The model under review builds one solid part; all positions refer to its coordinate system, in mm. Face numbers are marked on the shaded views. A direction names the side the tool comes from. Give positions to 0.01 mm unless a question says otherwise; leave off trailing zeros. Order: outer loops, then holes, each group sorted by start corner. A loop starts at its lowest first (then second) coordinate and runs counter-clockwise, first axis right, second up. Notation, with made-up numbers: (38.5, -9) -> (68.5, -9) arc R31 ccw to (68.5, 21) -> close; hole circle Ø10 at (-1.75, -16). An arc over 180 degrees is marked (long way). Use one line per item in the form item = value.
```python
from build123d import *

# Parameters (mm, degrees)
SKETCH1_W           = 71
SKETCH1_H           = 153
SKETCH1_W_2         = 65
SKETCH1_H_2         = 147
BOSS_EXTRUDE1_DEPTH = 10
SKETCH2_W           = 77
SKETCH2_H           = 159
SKETCH2_W_2         = 71
SKETCH2_H_2         = 153
BOSS_EXTRUDE2_DEPTH = 60
SKETCH3_W           = 71
SKETCH3_H           = 153
SKETCH3_W_2         = 65
SKETCH3_H_2         = 147
BOSS_EXTRUDE3_DEPTH = 10
RIB17_REACH         = 188.312
SKETCH7_WALL_W      = 379.62313401
SKETCH7_WALL_H      = 60
RIB22_REACH         = 188.312
SKETCH9_WALL_W      = 379.62313401
SKETCH9_WALL_H      = 60
RIB23_REACH         = 188.312
SKETCH10_WALL_W     = 379.62313401
SKETCH10_WALL_H     = 60
RIB24_REACH         = 188.312
SKETCH11_WALL_W     = 379.62313401
SKETCH11_WALL_H     = 60
FILLET1_R           = 2.5
FILLET2_R           = 3
SKETCH12_W          = 18
SKETCH12_H          = 8
CUT_EXTRUDE1_DEPTH  = 10
SKETCH13_W          = 12
SKETCH13_H          = 11
SKETCH13_W_2        = 25.5
SKETCH13_H_2        = 21.5
CUT_EXTRUDE2_DEPTH  = 10
SKETCH14_W          = 77
SKETCH14_H          = 159
CUT_EXTRUDE3_DEPTH  = 28.5
SKETCH15_W          = 71
SKETCH15_H          = 153
CUT_EXTRUDE4_DEPTH  = 5
FILLET3_R           = 2.5
SKETCH16_W          = 2
SKETCH16_H          = 11
BOSS_EXTRUDE4_DEPTH = 17
BOSS_EXTRUDE5_DEPTH = 11
SKETCH19_W          = 8
SKETCH19_H          = 2
BOSS_EXTRUDE7_DEPTH = 9
SKETCH20_W          = 8
SKETCH20_H          = 7
BOSS_EXTRUDE8_DEPTH = 3
SKETCH21_W          = 16
SKETCH21_H          = 2
BOSS_EXTRUDE9_DEPTH = 5
FILLET4_R           = 5


with BuildPart() as part:
    # Sketch1 → Boss-Extrude1 (new body)
    with BuildSketch(Plane(origin=(0, 0, 0), x_dir=(1, 0, 0), z_dir=(0, 1, 0))):
        with Locations((-35.5, 76.5)):
            Rectangle(SKETCH1_W, SKETCH1_H)
        with Locations((-35.5, 76.5)):
            Rectangle(SKETCH1_W_2, SKETCH1_H_2, mode=Mode.SUBTRACT)
    extrude(amount=BOSS_EXTRUDE1_DEPTH)



with BuildPart() as body_2:
    # Sketch2 → Boss-Extrude2 (new body)
    with BuildSketch(Plane(origin=(0, 10, 0), x_dir=(1, 0, 0), z_dir=(0, 1, 0))):
        with Locations((-35.5, 76.5)):
            Rectangle(SKETCH2_W, SKETCH2_H)
        with Locations((-35.5, 76.5)):
            Rectangle(SKETCH2_W_2, SKETCH2_H_2, mode=Mode.SUBTRACT)
    extrude(amount=BOSS_EXTRUDE2_DEPTH)


with BuildPart() as part_1:
    add(part.part)

    add(body_2.part)  # Boss-Extrude3 merges body 2
    # Sketch3 → Boss-Extrude3 (add)
    with BuildSketch(Plane(origin=(0, 10, 0), x_dir=(1, 0, 0), z_dir=(0, 1, 0))):
        with Locations((-35.5, 76.5)):
            Rectangle(SKETCH3_W, SKETCH3_H)
        with Locations((-35.5, 76.5)):
            Rectangle(SKETCH3_W_2, SKETCH3_H_2, mode=Mode.SUBTRACT)
    extrude(amount=BOSS_EXTRUDE3_DEPTH)

    # Sketch7 wall → Rib17 (add, up to next)
    with BuildSketch(Plane(origin=(-66.232233047, 0, -4.767766953), x_dir=(0.707106781187, 0, 0.707106781187), z_dir=(-0.707106781187, 0, 0.707106781187)), mode=Mode.PRIVATE) as rib17_sk1:
        with Locations((0, 30)):
            Rectangle(SKETCH7_WALL_W, SKETCH7_WALL_H)
    rib17_tool1 = extrude(rib17_sk1.sketch, amount=RIB17_REACH, mode=Mode.PRIVATE) - part_1.part
    add(rib17_tool1.solids().sort_by_distance((-66.232233047, 0, -4.767766953))[0])

    # Sketch9 wall → Rib22 (add, up to next)
    with BuildSketch(Plane(origin=(-66.232233047, 0, -148.232233047), x_dir=(0.707106781187, 0, -0.707106781187), z_dir=(0.707106781187, 0, 0.707106781187)), mode=Mode.PRIVATE) as rib22_sk1:
        with Locations((0, 30)):
            Rectangle(SKETCH9_WALL_W, SKETCH9_WALL_H)
    rib22_tool1 = extrude(rib22_sk1.sketch, amount=-RIB22_REACH, mode=Mode.PRIVATE) - part_1.part
    add(rib22_tool1.solids().sort_by_distance((-66.232233047, 0, -148.232233047))[0])

    # Sketch10 wall → Rib23 (add, up to next)
    with BuildSketch(Plane(origin=(-4.767766953, 0, -148.232233047), x_dir=(0.707106781187, 0, 0.707106781187), z_dir=(-0.707106781187, 0, 0.707106781187)), mode=Mode.PRIVATE) as rib23_sk1:
        with Locations((0, 30)):
            Rectangle(SKETCH10_WALL_W, SKETCH10_WALL_H)
    rib23_tool1 = extrude(rib23_sk1.sketch, amount=-RIB23_REACH, mode=Mode.PRIVATE) - part_1.part
    add(rib23_tool1.solids().sort_by_distance((-4.767766953, 0, -148.232233047))[0])

    # Sketch11 wall → Rib24 (add, up to next)
    with BuildSketch(Plane(origin=(-4.767766953, 0, -4.767766953), x_dir=(0.707106781187, 0, -0.707106781187), z_dir=(0.707106781187, 0, 0.707106781187)), mode=Mode.PRIVATE) as rib24_sk1:
        with Locations((0, 30)):
            Rectangle(SKETCH11_WALL_W, SKETCH11_WALL_H)
    rib24_tool1 = extrude(rib24_sk1.sketch, amount=RIB24_REACH, mode=Mode.PRIVATE) - part_1.part
    add(rib24_tool1.solids().sort_by_distance((-4.767766953, 0, -4.767766953))[0])

    # Fillet1
    fillet1_edges = [part_1.edges().sort_by_distance(p)[0] for p in [
        (0, 5, 0),
        (-71, 5, 0),
        (-71, 5, -153),
        (0, 5, -153),
    ]]
    fillet(fillet1_edges, radius=FILLET1_R)

    # Fillet2
    fillet2_edges = [part_1.edges().sort_by_distance(p)[0] for p in [
        (-71, 65, 0),
        (0, 65, 0),
        (0, 65, -153),
        (-71, 65, -153),
    ]]
    fillet(fillet2_edges, radius=FILLET2_R)

    # Sketch12 → Cut-Extrude1 (cut)
    with BuildSketch(Plane(origin=(0, 0, -156), x_dir=(-1, 0, 0), z_dir=(0, 0, -1))):
        with Locations((22, 14)):
            Rectangle(SKETCH12_W, SKETCH12_H)
        with Locations((49, 14)):
            Rectangle(SKETCH12_W, SKETCH12_H)
    extrude(amount=-CUT_EXTRUDE1_DEPTH, mode=Mode.SUBTRACT)

    # Sketch13 → Cut-Extrude2 (cut)
    with BuildSketch(Plane.ZY.offset(74)):
        Polygon((-47.45, 19.949747468), (-42.500252532, 15), (-25.999747468, 15), (-21.05, 19.949747468), (-21.05, 33.3), (-47.45, 33.3), align=None)
        with Locations((-73.45, 25.5)):
            Rectangle(SKETCH13_W, SKETCH13_H)
        with Locations((-102.2, 25.75)):
            Rectangle(SKETCH13_W_2, SKETCH13_H_2)
    extrude(amount=-CUT_EXTRUDE2_DEPTH, mode=Mode.SUBTRACT)

    # Sketch14 → Cut-Extrude3 (cut)
    with BuildSketch(Plane(origin=(0, 70, 0), x_dir=(1, 0, 0), z_dir=(0, 1, 0))):
        with Locations((-35.5, 76.5)):
            Rectangle(SKETCH14_W, SKETCH14_H)
    extrude(amount=-CUT_EXTRUDE3_DEPTH, mode=Mode.SUBTRACT)

    # Sketch15 → Cut-Extrude4 (cut)
    with BuildSketch(Plane(origin=(0, 41.5, 0), x_dir=(1, 0, 0), z_dir=(0, 1, 0))):
        with Locations((-35.5, 76.5)):
            Rectangle(SKETCH15_W, SKETCH15_H)
    extrude(amount=-CUT_EXTRUDE4_DEPTH, mode=Mode.SUBTRACT)

    # Fillet3
    fillet3_edges = [part_1.edges().sort_by_distance(p)[0] for p in [
        (-71, 39, 0),
        (-71, 39, -153),
        (0, 39, -153),
        (0, 39, 0),
    ]]
    fillet(fillet3_edges, radius=FILLET3_R)

    # Sketch16 → Boss-Extrude4 (add)
    with BuildSketch(Plane(origin=(-71, 0, 0), x_dir=(0, 0, -1), z_dir=(1, 0, 0))):
        with Locations((66.45, 25.5)):
            Rectangle(SKETCH16_W, SKETCH16_H)
        with Locations((80.45, 25.5)):
            Rectangle(SKETCH16_W, SKETCH16_H)
    extrude(amount=BOSS_EXTRUDE4_DEPTH)

    # Sketch17 → Boss-Extrude5 (add)
    with BuildSketch(Plane(origin=(0, 31, 0), x_dir=(1, 0, 0), z_dir=(0, 1, 0))):
        Polygon((-54, 79.45), (-56, 79.45), (-56, 77.45), (-54, 77.45), (-51, 79.45), (-51, 81.45), (-54, 81.45), align=None)
        Polygon((-56, 67.45), (-56, 69.45), (-54, 69.45), (-51, 67.45), (-51, 65.45), (-54, 65.45), (-54, 67.45), align=None)
    extrude(amount=-BOSS_EXTRUDE5_DEPTH)

    # Sketch19 → Boss-Extrude7 (add)
    with BuildSketch(Plane(origin=(-68, 0, 0), x_dir=(0, 0, -1), z_dir=(1, 0, 0))):
        with Locations((73.45, 19)):
            Rectangle(SKETCH19_W, SKETCH19_H)
    extrude(amount=BOSS_EXTRUDE7_DEPTH)

    # Sketch20 → Boss-Extrude8 (add)
    with BuildSketch(Plane.ZY.offset(74)):
        Polygon((-79.45, 31), (-77.45, 31), (-69.45, 31), (-67.45, 31), (-67.45, 20), (-69.45, 20), (-77.45, 20), (-79.45, 20), align=None)
        with Locations((-73.45, 25.5)):
            Rectangle(SKETCH20_W, SKETCH20_H, mode=Mode.SUBTRACT)
    extrude(amount=-BOSS_EXTRUDE8_DEPTH)

    # Sketch21 → Boss-Extrude9 (add)
    with BuildSketch(Plane(origin=(-71, 0, 0), x_dir=(0, 0, -1), z_dir=(1, 0, 0))):
        with Locations((73.45, 32)):
            Rectangle(SKETCH21_W, SKETCH21_H)
    extrude(amount=BOSS_EXTRUDE9_DEPTH)

    # Fillet4
    # the kernel refuses this fillet: 5 mm, written as the material it adds along each edge
    with BuildSketch(Plane(origin=(-68, 18, -77.45), x_dir=(0, -1, 0), z_dir=(0, 0, 1))) as fillet4_piece_1:
        with BuildLine():
            CenterArc((FILLET4_R, FILLET4_R), FILLET4_R, 180, 90)
            Line((0, FILLET4_R), (-FILLET4_R * 0.02, FILLET4_R))
            Line((-FILLET4_R * 0.02, FILLET4_R), (-FILLET4_R * 0.02, -FILLET4_R * 0.02))
            Line((-FILLET4_R * 0.02, -FILLET4_R * 0.02), (FILLET4_R, -FILLET4_R * 0.02))
            Line((FILLET4_R, -FILLET4_R * 0.02), (FILLET4_R, 0))
        make_face()
    extrude(amount=8)
    with BuildSketch(Plane(origin=(-71, 33, -81.45), x_dir=(0, 1, 0), z_dir=(0, 0, 1))) as fillet4_piece_2:
        with BuildLine():
            CenterArc((FILLET4_R, -FILLET4_R), FILLET4_R, 90, 90)
            Line((0, -FILLET4_R), (-FILLET4_R * 0.02, -FILLET4_R))
            Line((-FILLET4_R * 0.02, -FILLET4_R), (-FILLET4_R * 0.02, FILLET4_R * 0.02))
            Line((-FILLET4_R * 0.02, FILLET4_R * 0.02), (FILLET4_R, FILLET4_R * 0.02))
            Line((FILLET4_R, FILLET4_R * 0.02), (FILLET4_R, 0))
        make_face()
    extrude(amount=16)
    with BuildSketch(Plane(origin=(-71, 33, -81.45), x_dir=(0, 0, -1), z_dir=(0, -1, 0)), Plane(origin=(-71, 20, -65.45), x_dir=(0, 0, 1), z_dir=(0, 1, 0))) as fillet4_piece_3:
        with BuildLine():
            CenterArc((FILLET4_R, FILLET4_R), FILLET4_R, 180, 90)
            Line((0, FILLET4_R), (-FILLET4_R * 0.02, FILLET4_R))
            Line((-FILLET4_R * 0.02, FILLET4_R), (-FILLET4_R * 0.02, -FILLET4_R * 0.02))
            Line((-FILLET4_R * 0.02, -FILLET4_R * 0.02), (FILLET4_R, -FILLET4_R * 0.02))
            Line((FILLET4_R, -FILLET4_R * 0.02), (FILLET4_R, 0))
        make_face()
    extrude(amount=13)
    with BuildSketch(Plane(origin=(-71, 45.5, -81.45), x_dir=(0, 0, -1), z_dir=(0, -1, 0))) as fillet4_piece_4a_section:
        with BuildLine():
            CenterArc((FILLET4_R, FILLET4_R), FILLET4_R, 180, 90)
            Line((0, FILLET4_R), (-FILLET4_R * 0.02, FILLET4_R))
            Line((-FILLET4_R * 0.02, FILLET4_R), (-FILLET4_R * 0.02, -FILLET4_R * 0.02))
            Line((-FILLET4_R * 0.02, -FILLET4_R * 0.02), (FILLET4_R, -FILLET4_R * 0.02))
            Line((FILLET4_R, -FILLET4_R * 0.02), (FILLET4_R, 0))
        make_face()
    fillet4_piece_4a = extrude(amount=25.5, mode=Mode.PRIVATE)
    fillet4_piece_4a = split(fillet4_piece_4a, bisect_by=Plane(origin=(-69.868024429, 33, -82.581975571), z_dir=(0, 1, 0)), keep=Keep.TOP, mode=Mode.PRIVATE)
    with BuildSketch(Plane(origin=(-71, 33, -93.95), x_dir=(0, 1, 0), z_dir=(0, 0, 1))) as fillet4_piece_4b_section:
        with BuildLine():
            CenterArc((FILLET4_R, -FILLET4_R), FILLET4_R, 90, 90)
            Line((0, -FILLET4_R), (-FILLET4_R * 0.02, -FILLET4_R))
            Line((-FILLET4_R * 0.02, -FILLET4_R), (-FILLET4_R * 0.02, FILLET4_R * 0.02))
            Line((-FILLET4_R * 0.02, FILLET4_R * 0.02), (FILLET4_R, FILLET4_R * 0.02))
            Line((FILLET4_R, FILLET4_R * 0.02), (FILLET4_R, 0))
        make_face()
    fillet4_piece_4b = extrude(amount=28.5, mode=Mode.PRIVATE)
    fillet4_piece_4b = split(fillet4_piece_4b, bisect_by=Plane(origin=(-69.868024429, 34.131975571, -81.45), z_dir=(0, 0, -1)), keep=Keep.TOP, mode=Mode.PRIVATE)
    fillet4_piece_4 = fillet4_piece_4a & fillet4_piece_4b
    add(fillet4_piece_4)
    with BuildSketch(Plane(origin=(-71, 33, -81.45), x_dir=(0, 1, 0), z_dir=(0, 0, 1))) as fillet4_piece_5a_section:
        with BuildLine():
            CenterArc((FILLET4_R, -FILLET4_R), FILLET4_R, 90, 90)
            Line((0, -FILLET4_R), (-FILLET4_R * 0.02, -FILLET4_R))
            Line((-FILLET4_R * 0.02, -FILLET4_R), (-FILLET4_R * 0.02, FILLET4_R * 0.02))
            Line((-FILLET4_R * 0.02, FILLET4_R * 0.02), (FILLET4_R, FILLET4_R * 0.02))
            Line((FILLET4_R, FILLET4_R * 0.02), (FILLET4_R, 0))
        make_face()
    fillet4_piece_5a = extrude(amount=28.5, mode=Mode.PRIVATE)
    fillet4_piece_5a = split(fillet4_piece_5a, bisect_by=Plane(origin=(-69.868024429, 34.131975571, -65.45), z_dir=(0, 0, 1)), keep=Keep.TOP, mode=Mode.PRIVATE)
    with BuildSketch(Plane(origin=(-71, 20, -65.45), x_dir=(0, 0, 1), z_dir=(0, 1, 0))) as fillet4_piece_5b_section:
        with BuildLine():
            CenterArc((FILLET4_R, FILLET4_R), FILLET4_R, 180, 90)
            Line((0, FILLET4_R), (-FILLET4_R * 0.02, FILLET4_R))
            Line((-FILLET4_R * 0.02, FILLET4_R), (-FILLET4_R * 0.02, -FILLET4_R * 0.02))
            Line((-FILLET4_R * 0.02, -FILLET4_R * 0.02), (FILLET4_R, -FILLET4_R * 0.02))
            Line((FILLET4_R, -FILLET4_R * 0.02), (FILLET4_R, 0))
        make_face()
    fillet4_piece_5b = extrude(amount=25.5, mode=Mode.PRIVATE)
    fillet4_piece_5b = split(fillet4_piece_5b, bisect_by=Plane(origin=(-69.868024429, 33, -64.318024429), z_dir=(0, 1, 0)), keep=Keep.TOP, mode=Mode.PRIVATE)
    fillet4_piece_5 = fillet4_piece_5a & fillet4_piece_5b
    add(fillet4_piece_5)


solid = part_1.part
```
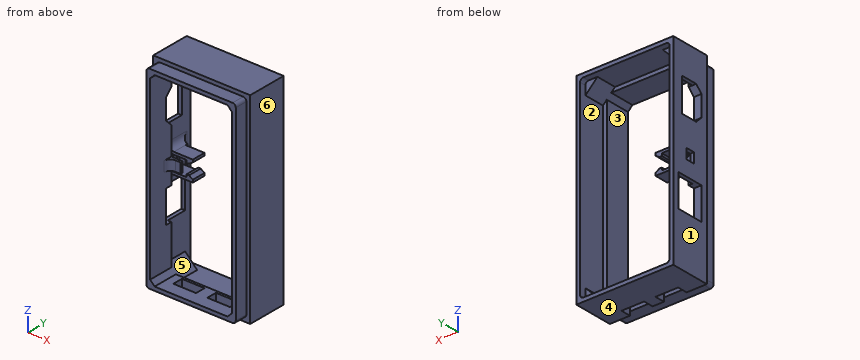
1. Add section D-D on z = -51. Give the boundary of the cut face in (x, y).
Values:
outline = (-74, 10) -> (-71, 10) -> (-71, 0) -> (-68, 0) -> (-68, 20) -> (-71, 20) -> (-71, 41.5) -> (-74, 41.5) -> close; (-3, 0) -> (0, 0) -> (0, 10) -> (3, 10) -> (3, 41.5) -> (0, 41.5) -> (0, 20) -> (-3, 20) -> close
2. For L1, parallel to Z at x = -59, y = 10.5; L2, parallel to X at y = 27, z = -122; L3, parallel to Z at x = -55, y = 28, list the stretches that pass through material, from the lowest coordinate up.
Values:
L1 = -156 to -150, -3 to 3
L2 = -74 to -71, 0 to 3
L3 = -156 to -153, -81.45 to -77.45, -69.45 to -65.45, 0 to 3
3. Add section A-A on z = -33. Give the boundary of the cut face in (x, y).
Values:
outline = (-74, 10) -> (-71, 10) -> (-71, 0) -> (-68, 0) -> (-68, 15) -> (-74, 15) -> close; (-74, 33.3) -> (-71, 33.3) -> (-71, 41.5) -> (-74, 41.5) -> close; (-3, 0) -> (0, 0) -> (0, 10) -> (3, 10) -> (3, 41.5) -> (0, 41.5) -> (0, 20) -> (-3, 20) -> close
4. Add section B-B on x = -34. Give the boundary of the cut face in (y, z), then the cut area to 3 significant figures.
Values:
outline = (0, -153) -> (10, -153) -> (10, -156) -> (41.5, -156) -> (41.5, -153) -> (20, -153) -> (20, -150) -> (0, -150) -> close; (0, -3) -> (20, -3) -> (20, 0) -> (41.5, 0) -> (41.5, 3) -> (10, 3) -> (10, 0) -> (0, 0) -> close
area = 309 mm^2
5. The part is to be moulded in two halves that separate along X. For the marked faces 4, 5 and 6, say which applies: +X half, -X half, draft (parallel to the pull), parting line (faces both ways), or undercut.
Values:
face_4 = draft
face_5 = undercut
face_6 = +X half
6. Add section C-C on y = 5.5. Give the boundary of the cut face in (x, z), then the cut area to 3 significant figures.
Values:
outline = (-71, -150.5) arc R2.5 ccw to (-68.5, -153) -> (-2.5, -153) arc R2.5 ccw to (0, -150.5) -> (0, -2.5) arc R2.5 ccw to (-2.5, 0) -> (-68.5, 0) arc R2.5 ccw to (-71, -2.5) -> close; hole (-68, -146.46) -> (-64.46, -150) -> (-6.54, -150) -> (-3, -146.46) -> (-3, -6.54) -> (-6.54, -3) -> (-64.46, -3) -> (-68, -6.54) -> close
area = 1,330 mm^2
7. Tool access review of the marked faces 1, 2 and 3: name each direction out of +Z, -Z, +X, -X, +Y, -Y from which nothing blocks a thin tool from reaching the whole face with its end or side.
Values:
face_1 = +Z, -Z, -X, +Y, -Y
face_2 = +Y
face_3 = +Y, -Y
8. For pin 1 Ø0.9 at (x, z) = (-34, -152) entering from +Y; pin 2 Ø6 at (x, y) = (-20.5, 12) entering from -Z; pin 3 Ø6 at (x, z) = (-8, -98.5) entering from -Y; pin 4 Ø3.5 at (x, z) = (-35, -155) entering from -Y, all flat-tipped, find the tip position at first contact; note any pin that passes through.
Values:
pin_1 = 20
pin_2 = -153
pin_3 = through
pin_4 = 10
